Geometry: final body of the model. Coordinates: model frame, mm. A direction names the side the tool comes from. Give positions to 0.01 mm unless a question says otherwise; leave off trailing zeros. Loops run counter-clockwise (first coordinate to the right, second up) from the corner with the lowest first, then second, coordinate; pieces in that order, holes last. Notation, with made-up numbers: M -35.5,-37 L -13.5,-37 A32 cw -13.5,-5 Z; hole C 30.5,45.25 d5. An arc over 180 degrees is marked long. One line per question, with ' | ' between items. Start each with the question number.
Autodesk Inventor part; units mm, degrees
ref_plane "YZ Plane" through (0, 0, 0) normal (1, 0, 0) x (0, 1, 0)
ref_plane "XZ Plane" through (0, 0, 0) normal (0, 1, 0) x (-1, 0, 0)
ref_plane "XY Plane" through (0, 0, 0) normal (0, 0, 1) x (1, 0, 0)
sketch "Sketch1" plane through (0, 0, 0) normal (0, 0, 1) x (1, 0, 0)
  circle A0 centre (0, 0) radius 6
  dimension "d0" = 12
extrude "Extrusion1" add sketch "Sketch1" along normal blind 69.85
sketch "Sketch2" plane through (0, 0, 69.85) normal (0, 0, 1) x (1, 0, 0)
  circle A0 centre (0, 0) radius 7.75
  dimension "d3" = 15.5
extrude "Extrusion2" add sketch "Sketch2" along normal blind 2.54
sketch "Sketch3" plane through (0, 0, 0) normal (0, 0, -1) x (-1, 0, 0)
  circle A0 centre (0, 0) radius 7.75
  dimension "d6" = 15.5
extrude "Extrusion3" add sketch "Sketch3" along normal blind 2.54
sketch "Sketch4" plane through (0, 0, 72.39) normal (0, 0, 1) x (1, 0, 0)
  circle A0 centre (0, 0) radius 2.5
  dimension "d9" = 5
extrude "Extrusion4" cut sketch "Sketch4" against normal blind 127
properties part number "SteelSpoolBar"
Q1. Contact query for flat-ended pins moving along their axis: pin 1 (2 mm diameter, centred on x = -3.5, z = 33.5, fed in from -Y); pin 2 (4 mm diameter, centred on x = -2.5, z = 6.5, fed in from +Y); pin 3 (2 mm diameter, centred on x = 3, z = 34.5, fed in from +Y). Output: stop coordinate, or through.
Q2. Section C-C, the plane z = 67. Output: boundary loops of the cut face in (x, y).
Q3. Section D-D, the plane y = -3.5. Output: boundary loops of the cut face in (x, z), plus the area to 3 significant figures.
Q4. Set-up query: faces 4 (the flat face through (-4, -5, 0)), 5 (the flat face through (-2, 2, 72.39)). Return all of +Z, -Z, +X, -X, +Y, -Y with unobstructed straight access to the full face (end or side cutting, diameter ignored); none if empty.
Q5. Section A-A, the plane x = 0. Output: boundary loops of the cut face in (y, z).
Q6. Material intervals for L1, parallel to Z at x = -6, y = -2; L2, parallel to Y at x = 0, z = 33; L3, parallel to X at y = -0.25, z = 3, sorted ascending.
Q7. Draft query along Z for faces 1 (the cylindrical face through (-1.009, -7.684, 71.102)), 2 (the flat face through (4, -5, 69.85)), 3 (the flat face through (2, 2, -2.54)). Return one class per face: released by +Z, released by -Z, zero draft, split by the parting line, or undercut.
Model answer:
1) pin 1: stops at y = -5.45 | pin 2: stops at y = 5.98 | pin 3: stops at y = 5.66
2) outline: C 0,0 d12; hole C 0,0 d5
3) outline: M -6.91,-2.54 L 6.91,-2.54 L 6.91,0 L 4.87,0 L 4.87,69.85 L 6.91,69.85 L 6.91,72.39 L -6.91,72.39 L -6.91,69.85 L -4.87,69.85 L -4.87,0 L -6.91,0 Z | area: 751 mm^2
4) face 4: none | face 5: +Z, +X, -X, +Y, -Y
5) outline: M -7.75,-2.54 L -2.5,-2.54 L -2.5,72.39 L -7.75,72.39 L -7.75,69.85 L -6,69.85 L -6,0 L -7.75,0 Z; M 2.5,-2.54 L 7.75,-2.54 L 7.75,0 L 6,0 L 6,69.85 L 7.75,69.85 L 7.75,72.39 L 2.5,72.39 Z
6) L1: z = -2.54 to 0, 69.85 to 72.39 | L2: y = -6 to -2.5, 2.5 to 6 | L3: x = -5.99 to -2.49, 2.49 to 5.99
7) face 1: zero draft | face 2: undercut | face 3: released by -Z
